Source: three-view drawing plus pictorial views. Frame: mm from the lowest corner of the part. Give positions to 0.01 mm unless a question says otherwise; leave off trailing zeros. Write each loop counter-clockwise with the first axis right and the second up, starting at its lowest first coordinate (ties: lowest second). Pieces come first, ordered by that corner, then holes.
Q1. Cut plane A-A on y = 105. Return the cut outline in (x, z) (3 decimals), plus the area to 3 significant figures.
Q2. Line query: L1, parallel to Y at x = 70.5, z = 0.9; L2, parallel to Y at x = 14, z = 0.5 (3 decimals); L3, parallel to X at y = 113.5, z = 1.45 (3 decimals). Output: solid intervals per line, ascending.
Q3. Cut plane B-B on x = 5. Return the cut outline in (y, z) (3 decimals).
Q4. Cut plane D-D on x = 38.1. Return the cut outline in (y, z) (3 decimals), plus the area to 3 significant figures.
Q5. Pin query (flat end, axial travel): pin 1 (1.6 mm diameter, centred on x = 4.5, z = 2, fed in from -Y). Return the tip coordinate at first contact, or that it passes through.
Q6. Cut plane C-C on z = 2.5. Count the separate pieces of the cut face and the enclosed holes in it, plus the area to 3 significant figures.
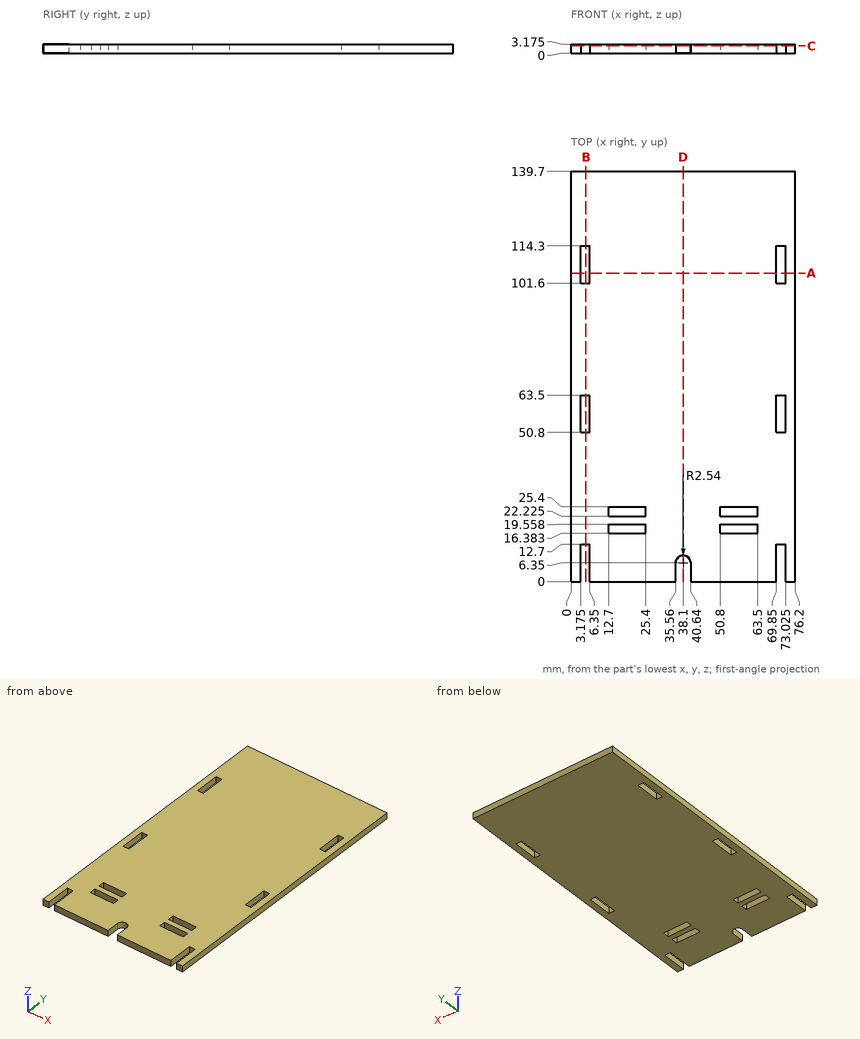
Data:
1. outline: (0, 0) - (3.175, 0) - (3.175, 3.175) - (0, 3.175) - close; (6.35, 0) - (69.85, 0) - (69.85, 3.175) - (6.35, 3.175) - close; (73.025, 0) - (76.2, 0) - (76.2, 3.175) - (73.025, 3.175) - close
1. area: 222 mm2
2. L1: y = 12.7 to 50.8, 63.5 to 101.6, 114.3 to 139.7
2. L2: y = 0 to 16.383, 19.558 to 22.225, 25.4 to 139.7
2. L3: x = 0 to 3.175, 6.35 to 69.85, 73.025 to 76.2
3. outline: (12.7, 0) - (50.8, 0) - (50.8, 3.175) - (12.7, 3.175) - close; (63.5, 0) - (101.6, 0) - (101.6, 3.175) - (63.5, 3.175) - close; (114.3, 0) - (139.7, 0) - (139.7, 3.175) - (114.3, 3.175) - close
4. outline: (8.89, 0) - (139.7, 0) - (139.7, 3.175) - (8.89, 3.175) - close
4. area: 415 mm2
5. pin 1: stops at y = 12.7
6. separate pieces: 1
6. enclosed holes: 8
6. area: 10,200 mm2
